Source: CAD feature listing. Evaluate the final solid. Frame: model axes, mm. Give positions to 0.01 mm unless a question says otherwise; leave off trailing zeros. Write each loop counter-clockwise with the first axis right and the second up, starting at its lowest first coordinate (ties: lowest second). Pieces come first, ordered by that corner, then holes. Notation, with made-up numbers: M 30.25,-14.5 L 49.25,-14.5 A6 ccw 49.25,-8.5 Z; hole C 75.25,79.25 d5. An arc over 180 degrees is marked long. Return JSON: item names as keys, results as strings.
```python
from build123d import *

# Parameters (mm, degrees)
F0_R     = 28.575
F0_R_2   = 12.6365
F1_DEPTH = 63.5
F4_DEPTH = 127


with BuildPart() as f1:
    # F0 (on Top) → F1 (new body, symmetric)
    with BuildSketch(Plane.XY):
        Circle(F0_R)
        with Locations((0, -12.7)):
            Circle(F0_R_2, mode=Mode.SUBTRACT)
        with Locations((0, 12.7)):
            Circle(F0_R_2, mode=Mode.SUBTRACT)
    extrude(amount=F1_DEPTH, both=True)

    # F3 (on offset) → F4 (cut)
    with BuildSketch(Plane.XY.offset(-63.5)):
        with BuildLine():
            ThreePointArc((15.8258405296, -23.792297), (18.3676559468, -21.8897199621), (20.6827101795, -19.716899468))
            ThreePointArc((20.6827101795, -19.716899468), (16.326805286, -19.4575288553), (15.8258405296, -23.792297))
        make_face()
        with BuildLine():
            ThreePointArc((24.3981417093, -14.8748548273), (25.8977450146, -12.0763168292), (27.0776230728, -9.1286884999))
            ThreePointArc((27.0776230728, -9.1286884999), (23.0202177907, -10.7345038482), (24.3981417093, -14.8748548273))
        make_face()
        with BuildLine():
            ThreePointArc((28.3986111111, -3.1700965222), (28.575, 0), (28.3986111111, 3.1700965222))
            ThreePointArc((28.3986111111, 3.1700965222), (25.4, 0), (28.3986111111, -3.1700965222))
        make_face()
        with BuildLine():
            ThreePointArc((27.0776230728, 9.1286884999), (25.8977450146, 12.0763168292), (24.3981417093, 14.8748548273))
            ThreePointArc((24.3981417093, 14.8748548273), (23.0202177907, 10.7345038482), (27.0776230728, 9.1286884999))
        make_face()
        with BuildLine():
            ThreePointArc((20.6827101795, 19.716899468), (18.3676559468, 21.8897199621), (15.8258405296, 23.792297))
            ThreePointArc((15.8258405296, 23.792297), (16.326805286, 19.4575288553), (20.6827101795, 19.716899468))
        make_face()
        with BuildLine():
            ThreePointArc((-20.6827101795, 19.716899468), (-16.326805286, 19.4575288553), (-15.8258405296, 23.792297))
            ThreePointArc((-15.8258405296, 23.792297), (-18.3676559468, 21.8897199621), (-20.6827101795, 19.716899468))
        make_face()
        with BuildLine():
            ThreePointArc((-27.0776230728, 9.1286884999), (-23.0202177907, 10.7345038482), (-24.3981417093, 14.8748548273))
            ThreePointArc((-24.3981417093, 14.8748548273), (-25.8977450146, 12.0763168292), (-27.0776230728, 9.1286884999))
        make_face()
        with BuildLine():
            ThreePointArc((-28.3986111111, -3.1700965222), (-25.4, 0), (-28.3986111111, 3.1700965222))
            ThreePointArc((-28.3986111111, 3.1700965222), (-28.575, 0), (-28.3986111111, -3.1700965222))
        make_face()
        with BuildLine():
            ThreePointArc((-24.3981417093, -14.8748548273), (-23.0202177907, -10.7345038482), (-27.0776230728, -9.1286884999))
            ThreePointArc((-27.0776230728, -9.1286884999), (-25.8977450146, -12.0763168292), (-24.3981417093, -14.8748548273))
        make_face()
        with BuildLine():
            ThreePointArc((-15.8258405296, -23.792297), (-16.326805286, -19.4575288553), (-20.6827101795, -19.716899468))
            ThreePointArc((-20.6827101795, -19.716899468), (-18.3676559468, -21.8897199621), (-15.8258405296, -23.792297))
        make_face()
    extrude(amount=F4_DEPTH, mode=Mode.SUBTRACT)


solid = f1.part
```
1) Cut plane D-D, the plane y = 11. Return the cut outline in (x, z), then the cut area to 3 significant figures.
Numbers:
{"outline": "M -22.91,-63.5 L -12.52,-63.5 L -12.52,63.5 L -22.91,63.5 Z; M 12.52,-63.5 L 22.91,-63.5 L 22.91,63.5 L 12.52,63.5 Z", "area": "2,640 mm²"}
2) Draft query along X for faces 1 (the face through (27.907, 6.143, 0.889)), 2 (the face through (-22.696, -17.361, 0.889)), 3 (the face through (12.05, -8.9, -0.89)), 4 (the face through (5.83, 1.49, -0.89)). Return one class per face: released by +X, released by -X, zero draft, split by the parting line, or undercut.
Numbers:
{"face 1": "released by +X", "face 2": "released by -X", "face 3": "undercut", "face 4": "undercut"}
3) Contact query for flat-ended pins moving along their axis: pin 1 Ø10 at (y, z) = (12.5, 17) entering from +X; pin 2 Ø4 at (x, z) = (10, 44) entering from -Y; pin 3 Ø2 at (x, z) = (2, -25.5) entering from -Y; pin 4 Ø20 at (x, y) = (0, 12.7) entering from +Z. Output: stop coordinate, or through.
Numbers:
{"pin 1": "stops at x = 27.57", "pin 2": "stops at y = -27.43", "pin 3": "stops at y = -28.56", "pin 4": "passes through"}
4) Cut plane C-C, the plane x = 8. Return the cut outline in (y, z), then the cut area to 3 significant figures.
Numbers:
{"outline": "M -27.43,-63.5 L -22.48,-63.5 L -22.48,63.5 L -27.43,63.5 Z; M -2.92,-63.5 L 2.92,-63.5 L 2.92,63.5 L -2.92,63.5 Z; M 22.48,-63.5 L 27.43,-63.5 L 27.43,63.5 L 22.48,63.5 Z", "area": "2,000 mm²"}
5) Cut plane B-B, the plane y = -6. Return the cut outline in (x, z).
Numbers:
{"outline": "M -27.94,-63.5 L -10.71,-63.5 L -10.71,63.5 L -27.94,63.5 Z; M 10.71,-63.5 L 27.94,-63.5 L 27.94,63.5 L 10.71,63.5 Z"}
6) Line query: line 1 (X direction, y = 12, z = 8); line 2 (Y direction, x = 10, z = 23.5); line 3 (Y direction, x = 1, z = 5). Output: solid intervals per line, ascending. Write a range as [from, to].
Numbers:
{"line 1": "x = [-22.72, -12.62], [12.62, 22.72]", "line 2": "y = [-26.77, -20.43], [-4.97, 4.97], [20.43, 26.77]", "line 3": "y = [-28.56, -25.3], [-0.1, 0.1], [25.3, 28.56]"}
7) Cut plane A-A, the plane x = 0. Give the number of separate pieces and of enclosed holes in the cut face, then the cut area to 3 significant figures.
Numbers:
{"separate pieces": "3", "enclosed holes": "0", "area": "839 mm²"}
